from build123d import *

# Parameters (mm, degrees)
SKETCH_3_R               = 12.9
EXTRUDE_1_DEPTH          = 9
EXTRUDE_2_DEPTH          = 5
SKETCH_5_R               = 6.1
EXTRUDE_3_DEPTH          = 2.5
SKETCH_6_R               = 4
CUT_EXTRUDE_1_DEPTH      = 29.370936
SKETCH_7_R               = 2.6
CUT_EXTRUDE_2_DEPTH      = 27.737801
CUT_EXTRUDE_3_DEPTH      = 17
CUT_EXTRUDE_3_DEPTH_BACK = 15
SKETCH_8_R               = 8


with BuildPart() as part:
    # 草图3 → 凸台-拉伸1 (new body)
    with BuildSketch(Plane(origin=(0, 0, 0), x_dir=(1, 0, 0), z_dir=(0, 1, 0))):
        with Locations(Location((0, 0, 0), (0, 0, 270))):
            Circle(SKETCH_3_R)
    extrude(amount=EXTRUDE_1_DEPTH)

    # 草图4 → 凸台-拉伸2 (add)
    with BuildSketch(Plane(origin=(0, 0, 0), x_dir=(1, 0, 0), z_dir=(0, 1, 0))):
        with BuildLine():
            Line((-20.424324, 3.506704), (-6.205946, 11.309122))
            ThreePointArc((-6.205946, 11.309122), (0, 12.9), (6.205946, 11.309122))
            Line((6.205946, 11.309122), (20.424324, 3.506704))
            ThreePointArc((20.424324, 3.506704), (22.5, 0), (20.424324, -3.506704))
            Line((20.424324, -3.506704), (6.205946, -11.309122))
            ThreePointArc((6.205946, -11.309122), (0, -12.9), (-6.205946, -11.309122))
            Line((-6.205946, -11.309122), (-20.424324, -3.506704))
            ThreePointArc((-20.424324, -3.506704), (-22.5, 0), (-20.424324, 3.506704))
        make_face()
    extrude(amount=EXTRUDE_2_DEPTH)

    # 草图5 → 凸台-拉伸3 (add)
    with BuildSketch(Plane(origin=(0, 9, 0), x_dir=(1, 0, 0), z_dir=(0, 1, 0))):
        with Locations(Location((0, 0, 0), (0, 0, 270))):
            Circle(SKETCH_5_R)
    extrude(amount=EXTRUDE_3_DEPTH)

    # 草图6 → 切除-拉伸1 (cut, through all)
    with BuildSketch(Plane(origin=(0, 11.5, 0), x_dir=(1, 0, 0), z_dir=(0, 1, 0))):
        with Locations(Location((0, 0, 0), (0, 0, 270))):
            Circle(SKETCH_6_R)
    extrude(amount=-CUT_EXTRUDE_1_DEPTH, mode=Mode.SUBTRACT)

    # 草图7 → 切除-拉伸2 (cut, through all)
    with BuildSketch(Plane(origin=(0, 5, 0), x_dir=(1, 0, 0), z_dir=(0, 1, 0))):
        with Locations(Location((18.5, 0, 0), (0, 0, 270))):
            Circle(SKETCH_7_R)
        with Locations(Location((-18.5, 0, 0), (0, 0, 270))):
            Circle(SKETCH_7_R)
    extrude(amount=-CUT_EXTRUDE_2_DEPTH, mode=Mode.SUBTRACT)

    # 草图8 → 切除-拉伸3 (cut, two sides: drawn at the far end of the back side and taken through both)
    with BuildSketch(Plane(origin=(0, 9, 0), x_dir=(1, 0, 0), z_dir=(0, 1, 0)).offset(-CUT_EXTRUDE_3_DEPTH_BACK)):
        with Locations(Location((0, 0, 0), (0, 0, 270))):
            Circle(SKETCH_8_R)
    extrude(amount=CUT_EXTRUDE_3_DEPTH + CUT_EXTRUDE_3_DEPTH_BACK, mode=Mode.SUBTRACT)


solid = part.part
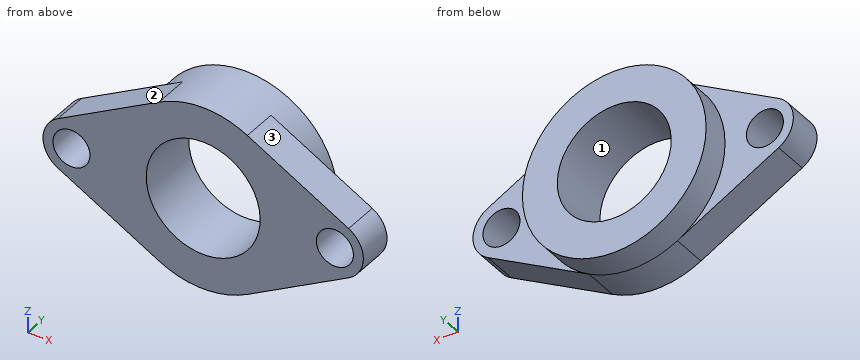
Verification items for the finished model (mm, model axes). Face numbers are marked on the shaded views. Give positions to 0.01 mm unless a question says otherwise; leave off trailing zeros. Write each loop counter-clockwise with the first axis right and the second up, starting at its lowest first coordinate (ties: lowest second). Pieces come first, ordered by that corner, then holes. Notation, with made-up numbers: M 3,41.5 L 10,41.5 A16 ccw 10,66.5 Z; hole C -7.75,-2 d10. An arc over 180 degrees is marked long. Write item = value, one per line.
(1) Sectioned sample at C-C (y = 3.25). Record the cut outline in (x, z).
Found:
outline = M -20.42,-3.51 L -6.21,-11.31 A12.9 ccw 6.21,-11.31 L 20.42,-3.51 A4 ccw 20.42,3.51 L 6.21,11.31 A12.9 ccw -6.21,11.31 L -20.42,3.51 A4 ccw Z; hole C -18.5,0 d5.2; hole C 0,0 d16; hole C 18.5,0 d5.2
(2) Sectioned sample at A-A (z = 0). Record the cut outline in (x, y).
Found:
outline = M -22.5,0 L -21.1,0 L -21.1,5 L -22.5,5 Z; M -15.9,0 L -8,0 L -8,9 L -12.9,9 L -12.9,5 L -15.9,5 Z; M 8,0 L 15.9,0 L 15.9,5 L 12.9,5 L 12.9,9 L 8,9 Z; M 21.1,0 L 22.5,0 L 22.5,5 L 21.1,5 Z
(3) Sectioned sample at D-D (z = -4). Record the cut outline in (x, y), then the cut area to 3 significant figures.
Found:
outline = M -19.53,0 L -6.93,0 L -6.93,9 L -12.26,9 L -12.26,5 L -19.53,5 Z; M 6.93,0 L 19.53,0 L 19.53,5 L 12.26,5 L 12.26,9 L 6.93,9 Z
area = 169 mm2
(4) Sectioned sample at B-B (x = 0). Record the cut outline in (y, z), then the cut area to 3 significant figures.
Found:
outline = M 0,-12.9 L 9,-12.9 L 9,-8 L 0,-8 Z; M 0,8 L 9,8 L 9,12.9 L 0,12.9 Z
area = 88.2 mm2
(5) Go/stop test with flat-tipped pins: pin 1 Ø4 at (x, y) = (9, 6.5) entering from -Z; pin 2 Ø3 at (y, z) = (7.5, -5) entering from +X; pin 3 Ø6 at (x, z) = (18.5, 0) entering from +Y. Record where each tip stops, or that it passes through.
Found:
pin_1 = -10.84
pin_2 = 12.42
pin_3 = 5
(6) Material ranges on line 1 (Y direction, x = -15, z = 4.25); line 2 (Z direction, x = 20, y = 2); line 3 (X direction, y = 8.5, z = -4.75), recorded low to high.
Found:
line_1 = 0 to 5
line_2 = -3.74 to -2.12, 2.12 to 3.74
line_3 = -11.99 to -6.44, 6.44 to 11.99
(7) Draft check along X on the marked faces 1, 2 and 3. Enter one of: released by +X, released by -X, zero draft, split by the parting line, or undercut.
Found:
face_1 = undercut
face_2 = released by -X
face_3 = released by +X
